```python
from build123d import *

# Parameters (mm, degrees)
BOSS_EXTRUDE1_DEPTH = 2.54


with BuildPart() as part:
    # Sketch2 → Boss-Extrude1 (new body)
    with BuildSketch(Plane.XY):
        with BuildLine():
            Line((52.480544155, 258.674987582), (196.894837031, 296.342844243))
            Line((196.894837031, 296.342844243), (206.373128662, 291.523930207))
            Line((206.373128662, 291.523930207), (216.178620917, 257.355486833))
            ThreePointArc((216.178620917, 257.355486833), (218.633828258, 242.895591751), (217.836941691, 228.250402074))
            Line((217.836941691, 228.250402074), (213.120538575, 200.036424744))
            ThreePointArc((213.120538575, 200.036424744), (196.554033533, 156.731222664), (164.448728673, 123.279182124))
            Line((164.448728673, 123.279182124), (133.560538269, 101.865242067))
            ThreePointArc((133.560538269, 101.865242067), (73.755681182, 87.130889432), (19.343587989, 115.99342905))
            Line((19.343587989, 115.99342905), (18.948822289, 116.444928865))
            ThreePointArc((18.948822289, 116.444928865), (7.419590663, 136.102703369), (3.91533799, 158.620951381))
            Line((3.91533799, 158.620951381), (5.226431104, 197.573753427))
            ThreePointArc((5.226431104, 197.573753427), (18.98894665, 235.75335118), (52.480544155, 258.674987582))
        make_face()
    extrude(amount=BOSS_EXTRUDE1_DEPTH)


solid = part.part
```
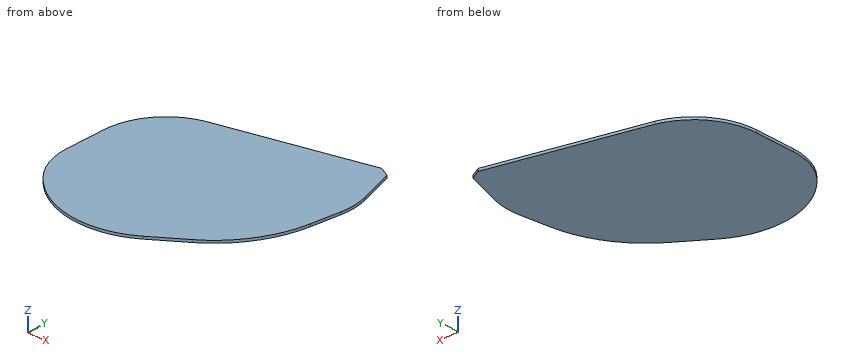
Can you work these out from the model? Positions are in its coordinate system, mm. Round coordinates to 2 decimals unless told otherwise and drop trailing zeros. Order: outer loops, then holes, each group sorted by start corner. A loop starts at its lowest first (then second) coordinate and runs counter-clockwise, first axis right, second up. Notation, with made-up numbers: (-30.5, 14.25) -> (5.5, 14.25) arc R24 cw to (5.5, 35.25) -> close; hole circle Ø6 at (-4, 64.5). An arc over 180 degrees is marked (long way). Return JSON: item names as keys, results as strings. Group by question number.
1. If we section it at B-B, the plane y = 164: Write out the boundary of the cut face in (x, z).
2. If we section it at C-C, the plane x = 85: Write out the boundary of the cut face in (y, z).
3. If we section it at A-A, the plane z = 1.35: Write out the boundary of the cut face in (x, y), then the cut area to 3 significant figures.
4. I need wall thicknesses on line 1 (Y direction, x = 180.5, z = 1.05); line 2 (X direction, y = 211, z = 2.4); line 3 (Y direction, x = 204.5, z = 1.45). Which ranges of each line are inside material? Lowest first, please. Write a range as [from, to].
5. Will this pin go through, and if not, where does the flat tip stop? pin 1 (2 mm diameter, centred on x = 139.5, y = 143, fed in from -Z).
Output values:
{
 "1": {"outline": "(4.1, 0) -> (200.8, 0) -> (200.8, 2.54) -> (4.1, 2.54) -> close"},
 "2": {"outline": "(86.48, 0) -> (267.16, 0) -> (267.16, 2.54) -> (86.48, 2.54) -> close"},
 "3": {"outline": "(3.92, 158.62) arc R60.96 ccw to (18.95, 116.44) -> (19.34, 115.99) arc R86.36 ccw to (133.56, 101.87) -> (164.45, 123.28) arc R116.84 ccw to (213.12, 200.04) -> (217.84, 228.25) arc R66.04 ccw to (216.18, 257.36) -> (206.37, 291.52) -> (196.89, 296.34) -> (52.48, 258.67) arc R66.04 ccw to (5.23, 197.57) -> close", "area": "33,200 mm²"},
 "4": {"line 1": "[136.68, 292.07]", "line 2": "[7.07, 214.95]", "line 3": "[171.51, 292.48]"},
 "5": {"pin 1": "z = 0"}
}
